Part print with two shaded views. Sizes in mm from the minimum x, y, z corner. A direction names the side the tool comes from. Round coordinates to 2 decimals unless told otherwise and drop trailing zeros. Order: outer loops, then holes, each group sorted by start corner. A loop starts at its lowest first (then second) coordinate and runs counter-clockwise, first axis right, second up. Notation, with made-up numbers: (11, 57.5) -> (17, 57.5) arc R36 ccw to (17, 92.5) -> close; hole circle Ø7 at (73, -39.5). An arc over 180 degrees is marked (long way). Use a Markdown table: item, result. Add a question column.
Item 1: Slice it at B-B, the plane z = 25.5. Give the cut face in (x, y), plus the area to 3 significant figures.
Item 2: Two-plate mould, pull along Y, no slides. Class the marked faces 3 and 4: released by +Y, released by -Y, zero draft, split by the parting line, or undercut.
Item 3: Slice it at C-C, the plane y = 4. Give the cut face in (x, z), plus the area to 4 significant figures.
Item 4: Slice it at A-A, the plane x = 39. Give the cut face in (y, z), plus the area to 3 significant figures.
Item 5: Pin check, flat tips, straight feed: pin 1 (11.5 mm diameter, centred on x = 22, y = 7.5, fed in from +Z); pin 2 (1 mm diameter, centred on y = 12.5, z = 23.5, fed in from +X); pin 3 (0.8 mm diameter, centred on y = 18.5, z = 27.5, fed in from +X); pin 4 (6 mm diameter, centred on x = 21.5, z = 18.5, fed in from -Y). Stop position of each tip, or through.
Item 6: Probe L1, parallel to Z at x = 27, y = 7.5; L2, parallel to Y at x = 16, z = 6.5; L3, parallel to Y at x = 36, z = 25.25. List the from-to ranges inside material, lowest first.
Item 7: 3-axis set-ups, long thin cutter, end or side, ignore diameter. For the marked faces 1 and 2: which of +Z, -Z, +X, -X, +Y, -Y reach the whole face in a straight line?
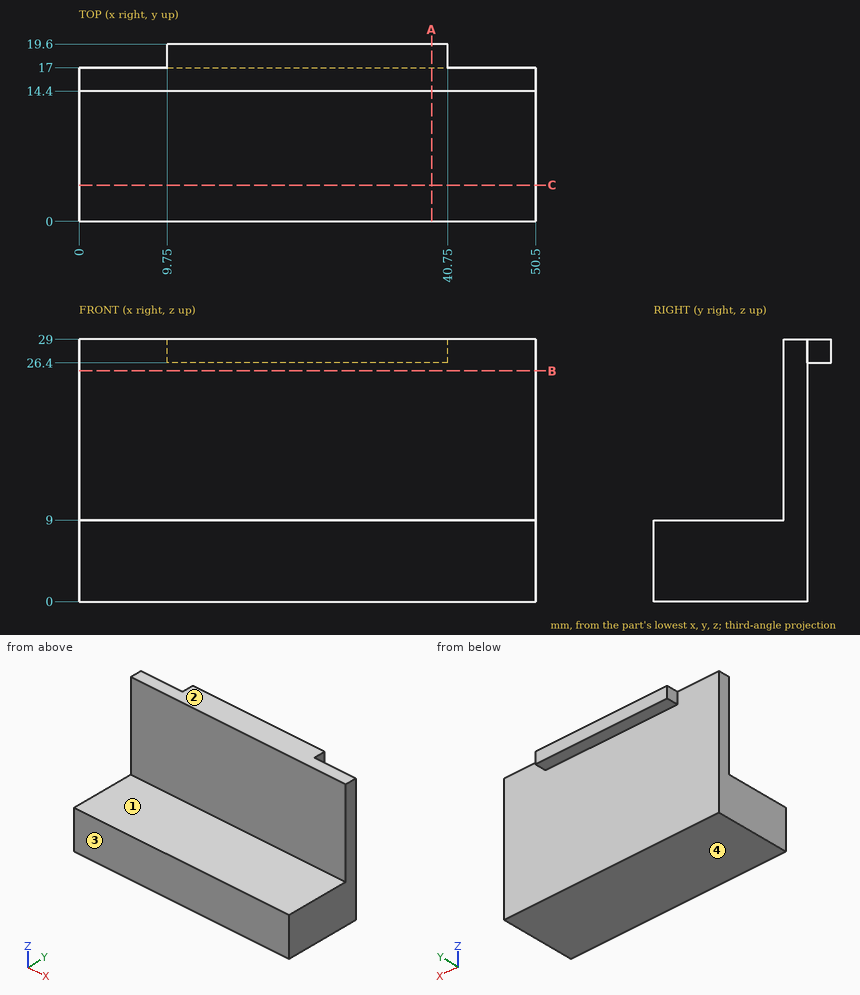
Check sheet entries:
| question | item | result |
|---|---|---|
| 1 | outline | (0, 14.4) -> (50.5, 14.4) -> (50.5, 17) -> (0, 17) -> close |
| 1 | area | 131 mm2 |
| 2 | face 3 | released by -Y |
| 2 | face 4 | zero draft |
| 3 | outline | (0, 0) -> (50.5, 0) -> (50.5, 9) -> (0, 9) -> close |
| 3 | area | 454.5 mm2 |
| 4 | outline | (0, 0) -> (17, 0) -> (17, 26.4) -> (19.6, 26.4) -> (19.6, 29) -> (14.4, 29) -> (14.4, 9) -> (0, 9) -> close |
| 4 | area | 212 mm2 |
| 5 | pin 1 | z = 9 |
| 5 | pin 2 | through |
| 5 | pin 3 | x = 40.75 |
| 5 | pin 4 | y = 14.4 |
| 6 | L1 | 0 to 9 |
| 6 | L2 | 0 to 17 |
| 6 | L3 | 14.4 to 17 |
| 7 | face 1 | +Z, +X, -X, -Y |
| 7 | face 2 | +Z, +X, -X, +Y, -Y |
